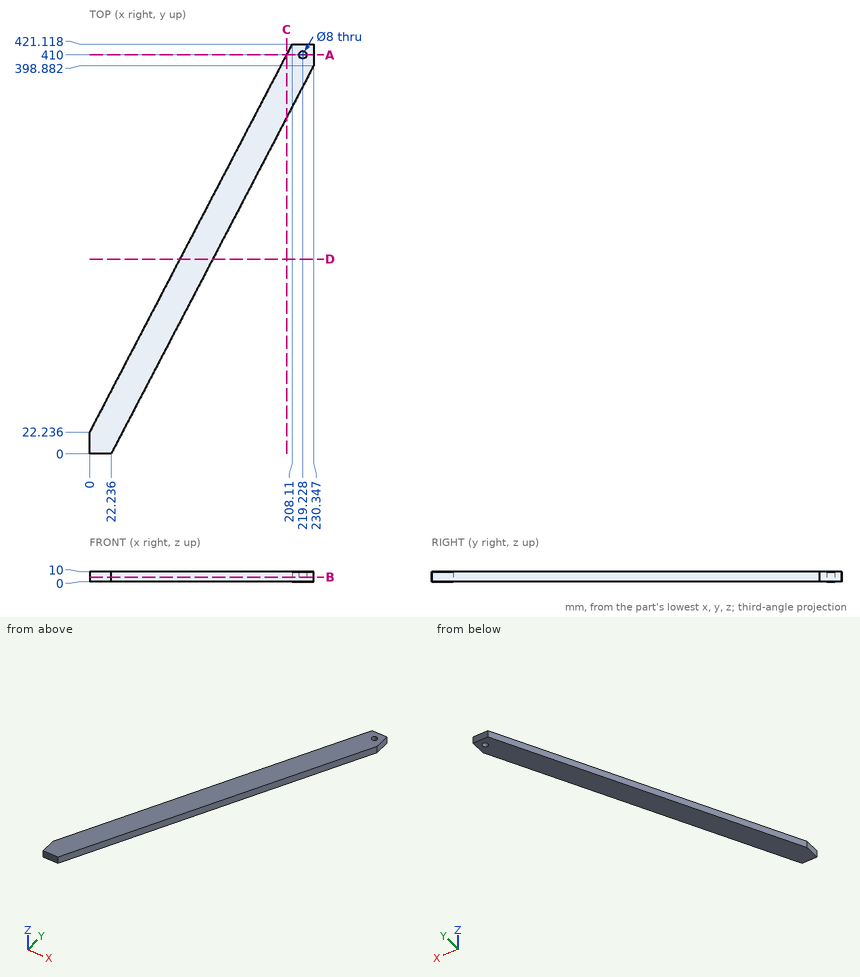
The figure shows three views and two pictorial views of one solid part (mm, origin at its lowest corner). Answer the questions. Coordinates: 2 decimals unless noted, no trailing zeros. Order: outer loops, then holes, each group sorted by start corner. A loop starts at its lowest first (then second) coordinate and runs counter-clockwise, first axis right, second up.
Q1. Given P1, Ø5, axis at y = 319.5, z = 8.5, coming from the +X side (1 decimal); P2, Ø4, axis at x = 50, z = 5.5, coming from the +Y side (1 decimal); P3, Ø1, axis at x = 183.5, z = 1, coming from the -Y side (1 decimal), each flat-ended and moving along its own axis, determine where each tip first touches the part or whether it passes through.
Q2. A cutting plane is placed at D-D, the plane y = 200. Write down the section's boundary in (x, z) (1 decimal).
Q3. A cutting plane is placed at B-B, the plane z = 4.5. Write down the section's boundary in (x, y).
Q4. Consider line 1 (X direction, y = 410, z = 5) (1 decimal); line 2 (X direction, y = 212, z = 3.5) (1 decimal); line 3 (Y direction, x = 34.5, z = 3.25) (1 decimal). Determine where each line is inside the solid, lowest interval first.
Q5. A cutting plane is placed at C-C, the plane x = 202.5. Write down the section's boundary in (y, z) (1 decimal).
Q6. A cutting plane is placed at A-A, the plane y = 410. Write down the section's boundary in (x, z).
Answers follow:
1. P1: stops at x = 190.2
1. P2: stops at y = 121.9
1. P3: stops at y = 308.1
2. outline: (92.7, 0) - (126.6, 0) - (126.6, 10) - (92.7, 10) - close
3. outline: (0, 0) - (22.24, 0) - (230.35, 398.88) - (230.35, 421.12) - (208.11, 421.12) - (0, 22.24) - close; hole circle Ø8 at (219.23, 410)
4. line 1: x = 202.3 to 215.2, 223.2 to 230.3
4. line 2: x = 99 to 132.8
4. line 3: y = 23.5 to 88.4
5. outline: (345.5, 0) - (410.4, 0) - (410.4, 10) - (345.5, 10) - close
6. outline: (202.31, 0) - (215.23, 0) - (215.23, 10) - (202.31, 10) - close; (223.23, 0) - (230.35, 0) - (230.35, 10) - (223.23, 10) - close
